Could you check a few things on this model? Use its own coordinates, in mm. Face numbers are marked on the shaded views. A direction names the side the tool comes from. Give positions to 0.01 mm unless a question says otherwise; leave off trailing zeros. Loops run counter-clockwise (first coordinate to the right, second up) from the corner with the lowest first, then second, coordinate; pieces in that order, holes last. Notation, with made-up numbers: (6.25, 29.5) - (65.25, 29.5) arc R14 ccw to (65.25, 53.5) - close; hole circle Ø1 at (-7.75, -13). An arc over 180 degrees is marked (long way). Write each question's results on one line, items separated by ' | '. Start each with the question number.
1) On a 3-axis mill with a long thin cutter (end or side, diameter ignored), from which of +Z, -Z, +X, -X, +Y, -Y can I reach the whole of each face in a straight line? I mean the marked faces 1 and 2. Say none if no direction works.
2) I want a section at A-A, the plane z = 17. Write out the boundary of the cut face in (x, y), and give its area (3 significant figures).
3) If we mould it in two halves opening along Y, with no side actions, what happens to the marked faces 3, 4 and 5? For each: +Y half, -Y half, draft (parallel to the pull), parting line (faces both ways), or undercut.
4) I want a section at C-C, the plane y = -7. Write out the boundary of the cut face in (x, z), and give its area (3 significant figures).
5) I'm going to push flat-ended pins straight in: pin 1 (14 mm diameter, centred on x = 1, z = -14.5, fed in from +Y); pin 2 (6.5 mm diameter, centred on x = -1, y = -0.5, fed in from +Z); pin 3 (5.5 mm diameter, centred on y = 102.5, z = -15.5, fed in from -X); pin 4 (5 mm diameter, centred on x = 14, z = -6, fed in from -Y). Where does each tip first touch, or does it pass through?
6) If I drill on probe 1 along Y at (x, z) = (0, 15); probe 2 along Y at (x, z) = (0, 20); probe 3 along X at (y, z) = (110, 0), over which ranges is the centre line in solid material (lowest first)? Write a range as [from, to].
7) I want a section at B-B, the plane z = -15.5. Write out the boundary of the cut face in (x, y), and give its area (3 significant figures).
8) I want a section at D-D, the plane z = 4.5. Write out the boundary of the cut face in (x, y), and give its area (3 significant figures).
from build123d import *

# Parameters (mm, degrees)
BOSS_EXTRUDE1_DEPTH = 21.5
SKETCH2_R           = 10.75
CUT_EXTRUDE1_DEPTH  = 2.5
SKETCH3_R           = 3
SKETCH3_R_2         = 1.6
CUT_EXTRUDE2_DEPTH  = 10
SKETCH4_R           = 4
BOSS_EXTRUDE2_DEPTH = 6
SKETCH6_W           = 12.8
SKETCH6_H           = 23.5
CUT_EXTRUDE3_DEPTH  = 18
SKETCH8_R           = 1
CUT_EXTRUDE4_DEPTH  = 8


with BuildPart() as part:
    # Sketch1 → Boss-Extrude1 (new, symmetric)
    with BuildSketch(Plane.XY):
        with BuildLine():
            Line((16, 110), (24.685901916, 0))
            ThreePointArc((24.685901916, 0), (0, -24.685901916), (-24.685901916, 0))
            Line((-24.685901916, 0), (-16, 110))
            ThreePointArc((-16, 110), (0, 126), (16, 110))
        make_face()
    extrude(amount=BOSS_EXTRUDE1_DEPTH, both=True)

    # Sketch2 → Cut-Extrude1 (cut)
    with BuildSketch(Plane.XY.offset(21.5)):
        Circle(SKETCH2_R)
    extrude(amount=-CUT_EXTRUDE1_DEPTH, mode=Mode.SUBTRACT)

    # Sketch3 → Cut-Extrude2 (cut)
    with BuildSketch(Plane.XY.offset(19)):
        Circle(SKETCH3_R)
        with Locations((0, 7)):
            Circle(SKETCH3_R_2)
        with Locations((7, 0)):
            Circle(SKETCH3_R_2)
        with Locations((0, -7)):
            Circle(SKETCH3_R_2)
        with Locations((-7, 0)):
            Circle(SKETCH3_R_2)
    extrude(amount=-CUT_EXTRUDE2_DEPTH, mode=Mode.SUBTRACT)

    # Sketch4 → Boss-Extrude2 (add)
    with BuildSketch(Plane(origin=(0, 0, -21.5), x_dir=(-1, 0, 0), z_dir=(0, 0, -1))):
        Circle(SKETCH4_R)
    extrude(amount=BOSS_EXTRUDE2_DEPTH)

    # Sketch6 → Cut-Extrude3 (cut)
    with BuildSketch(Plane(origin=(0, 0, -21.5), x_dir=(-1, 0, 0), z_dir=(0, 0, -1))):
        with Locations((0, 104.25)):
            Rectangle(SKETCH6_W, SKETCH6_H)
    extrude(amount=-CUT_EXTRUDE3_DEPTH, mode=Mode.SUBTRACT)

    # Sketch8 → Cut-Extrude4 (cut)
    with BuildSketch(Plane(origin=(0, 0, -21.5), x_dir=(-1, 0, 0), z_dir=(0, 0, -1))):
        with Locations((0, 118.6)):
            Circle(SKETCH8_R)
        with Locations((0, 89.9)):
            Circle(SKETCH8_R)
    extrude(amount=-CUT_EXTRUDE4_DEPTH, mode=Mode.SUBTRACT)


solid = part.part
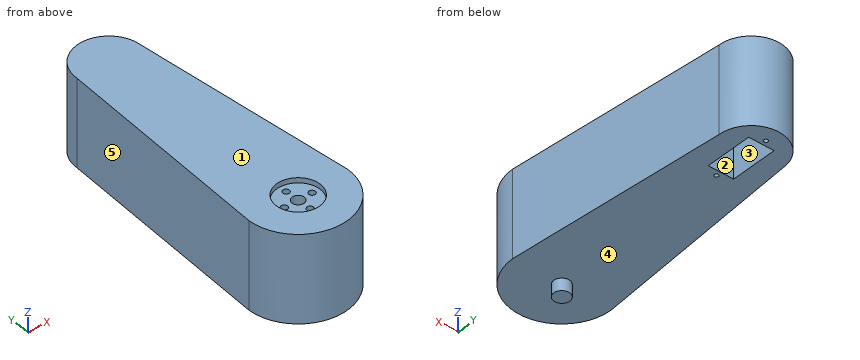
Answers:
1) face 1: +Z, +X, -X, +Y, -Y | face 2: -Z
2) outline: (-24.69, 0) arc R24.69 ccw to (24.69, 0) - (16, 110) arc R16 ccw to (-16, 110) - close; hole circle Ø3.2 at (-7, 0); hole circle Ø6 at (0, 0); hole circle Ø3.2 at (0, -7); hole circle Ø3.2 at (0, 7); hole circle Ø3.2 at (7, 0) | area: 5,770 mm2
3) face 3: undercut | face 4: draft | face 5: +Y half
4) outline: (-23.67, -21.5) - (23.67, -21.5) - (23.67, 21.5) - (8.16, 21.5) - (8.16, 19) - (1.6, 19) - (1.6, 9) - (-1.6, 9) - (-1.6, 19) - (-8.16, 19) - (-8.16, 21.5) - (-23.67, 21.5) - close | area: 1,960 mm2
5) pin 1: stops at y = 126 | pin 2: stops at z = 19 | pin 3: stops at x = -16.81 | pin 4: stops at y = -21.84
6) probe 1: y = [-24.69, -8.6], [-5.4, -3], [3, 5.4], [8.6, 126] | probe 2: y = [-24.69, -10.75], [10.75, 126] | probe 3: x = [-16, 16]
7) outline: (-24.69, 0) arc R24.69 ccw to (24.69, 0) - (16, 110) arc R16 ccw to (-16, 110) - close; hole (-6.4, 92.5) - (6.4, 92.5) - (6.4, 116) - (-6.4, 116) - close; hole circle Ø2 at (0, 89.9); hole circle Ø2 at (0, 118.6) | area: 5,530 mm2
8) outline: (-24.69, 0) arc R24.69 ccw to (24.69, 0) - (16, 110) arc R16 ccw to (-16, 110) - close | area: 5,830 mm2
